Design review of the part built by this model. Coordinates are the model's own, in mm. Face numbers are marked on the shaded views. A direction names the side the tool comes from. Coordinates: 2 decimals unless noted, no trailing zeros. Loops run counter-clockwise (first coordinate to the right, second up) from the corner with the lowest first, then second, coordinate; pieces in that order, holes last. Notation, with made-up numbers: M -30.5,78 L -18.5,78 A12 ccw -18.5,92 Z; hole C 25,45 d5. An arc over 180 degrees is marked long. One line per item, written item: value.
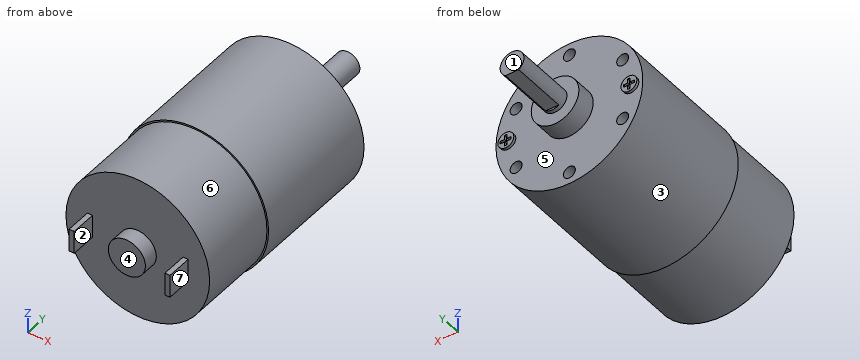
```python
from build123d import *

# Parameters (mm, degrees)
SKETCH1_R                 = 18.1
BASE_EXTRUDE_DEPTH        = 20
SKETCH2_R                 = 18.5
MOTOR_TOP_DEPTH           = 33.3
SKETCH3_R                 = 4.666403254
REAR_NUB_DEPTH            = 3.81
SKETCH4_W                 = 1.27
SKETCH4_H                 = 5.788702771
TEETH_PLUGS_DEPTH         = 6.35
SKETCH5_R                 = 6
AXLE_BASE_DEPTH           = 5
SKETCH7_R                 = 3
AXLE_DEPTH                = 15
SKETCH8_W                 = 0.5
SKETCH8_H                 = 14
D_SHAFT_CUTOUT_DEPTH      = 19.5
D_SHAFT_CUTOUT_DEPTH_BACK = 19.5
SKETCH9_R                 = 1.5
M3_SCREW_HOLES_DEPTH      = 10
SCREW_HOLE_PATTERN_COUNT  = 6
SKETCH10_R                = 2
PHILIPS_SCREWS_DEPTH      = 0.7


with BuildPart() as part:
    # Sketch1 → Base Extrude (new body)
    with BuildSketch(Plane(origin=(0, 0, 0), x_dir=(1, 0, 0), z_dir=(0, 1, 0))):
        Circle(SKETCH1_R)
    extrude(amount=BASE_EXTRUDE_DEPTH)

    # Sketch2 → Motor Top (add)
    with BuildSketch(Plane(origin=(0, 20, 0), x_dir=(1, 0, 0), z_dir=(0, 1, 0))):
        Circle(SKETCH2_R)
    extrude(amount=MOTOR_TOP_DEPTH)

    # Sketch3 → Rear nub (add)
    with BuildSketch(Plane.XZ):
        Circle(SKETCH3_R)
    extrude(amount=REAR_NUB_DEPTH)

    # Sketch4 → Teeth plugs (add)
    with BuildSketch(Plane.XZ):
        with Locations((-12.065, 0.236273582)):
            Rectangle(SKETCH4_W, SKETCH4_H)
        with Locations((12.065, 0.236273582)):
            Rectangle(SKETCH4_W, SKETCH4_H)
    extrude(amount=TEETH_PLUGS_DEPTH)

    # Sketch5 → Axle base (add)
    with BuildSketch(Plane(origin=(0, 53.3, 0), x_dir=(1, 0, 0), z_dir=(0, 1, 0))):
        Circle(SKETCH5_R)
    extrude(amount=AXLE_BASE_DEPTH)

    # Sketch7 → Axle (add)
    with BuildSketch(Plane(origin=(0, 58.3, 0), x_dir=(1, 0, 0), z_dir=(0, 1, 0))):
        Circle(SKETCH7_R)
    extrude(amount=AXLE_DEPTH)

    # Sketch8 → D shaft cutout (cut, two sides)
    with BuildSketch(Plane(origin=(0, 0, 0), x_dir=(0, 0, -1), z_dir=(1, 0, 0))) as d_shaft_cutout_sk:
        with Locations((2.75, 66.3)):
            Rectangle(SKETCH8_W, SKETCH8_H)
    extrude(amount=D_SHAFT_CUTOUT_DEPTH, mode=Mode.SUBTRACT)
    extrude(d_shaft_cutout_sk.sketch, amount=-D_SHAFT_CUTOUT_DEPTH_BACK, mode=Mode.SUBTRACT)

    # Sketch9 → M3 Screw Holes (cut)
    with BuildSketch(Plane(origin=(0, 53.3, 0), x_dir=(1, 0, 0), z_dir=(0, 1, 0))):
        with Locations((0, 15.5)):
            Circle(SKETCH9_R)
    m3_screw_holes = extrude(amount=-M3_SCREW_HOLES_DEPTH, mode=Mode.SUBTRACT)

    # Screw Hole Pattern: M3 Screw Holes ×6 about axis
    screw_hole_pattern_axis = Axis((0, 0, 0), (0, 1, 0))
    for i in range(1, SCREW_HOLE_PATTERN_COUNT):
        add(m3_screw_holes.rotate(screw_hole_pattern_axis, i * 360 / SCREW_HOLE_PATTERN_COUNT), mode=Mode.SUBTRACT)

    # Sketch10 → Philips Screws (add)
    with BuildSketch(Plane(origin=(0, 53.3, 0), x_dir=(1, 0, 0), z_dir=(0, 1, 0))):
        with Locations((-15.5, 0)):
            Circle(SKETCH10_R)
        Polygon((-16.943750133, -0.329942757), (-16.943750133, 0.329942757), (-15.829942757, 0.329942757), (-15.829942757, 1.40634253), (-15.170057243, 1.40634253), (-15.170057243, 0.329942757), (-14.166731925, 0.329942757), (-14.166731925, -0.329942757), (-15.170057243, -0.329942757), (-15.170057243, -1.370675678), (-15.829942757, -1.370675678), (-15.829942757, -0.329942757), align=None, mode=Mode.SUBTRACT)
        with Locations((15.5, 0)):
            Circle(SKETCH10_R)
        Polygon((15.829942757, 0.329942757), (16.943750133, 0.329942757), (16.943750133, -0.329942757), (15.829942757, -0.329942757), (15.829942757, -1.370675678), (15.170057243, -1.370675678), (15.170057243, -0.329942757), (14.166731925, -0.329942757), (14.166731925, 0.329942757), (15.170057243, 0.329942757), (15.170057243, 1.40634253), (15.829942757, 1.40634253), align=None, mode=Mode.SUBTRACT)
    extrude(amount=PHILIPS_SCREWS_DEPTH)


solid = part.part
```
(1) Tool access review of the marked faces 4, 5, 6 and 7: name each direction out of +Z, -Z, +X, -X, +Y, -Y from which nothing blocks a thin tool from reaching the whole face with its end or side.
Reply:
face 4: +Z, -Z, -Y
face 5: +Y
face 6: -Y
face 7: +Z, -Z, +X, -Y
(2) To check wall thickness, follow line 1 along Z through (x, y) = (0, 48.5); line 2 along Y through (x, z) = (6, 6); line 3 along X through (y, z) = (52.5, 8). State the ranges of each line that lie inside material, in increasing order. Write a range as [from, to].
Reply:
line 1: z = [-18.5, -17], [-14, 14], [17, 18.5]
line 2: y = [0, 53.3]
line 3: x = [-16.68, -14.9], [-11.94, 11.94], [14.9, 16.68]
(3) Insertion check: pin 1 (6 mm diameter, centred on y = 12, z = -10.5, fed in from +X); pin 2 (1 mm diameter, centred on y = 6.5, z = -1, fed in from -X); pin 3 (3.5 mm diameter, centred on x = -13, z = -8.5, fed in from +Y). Each pin has a flat end and moves straight along its axis. Give the tip position at first contact, or say it passes through.
Reply:
pin 1: stops at x = 16.47
pin 2: stops at x = -18.09
pin 3: stops at y = 53.3
(4) Mouldability with a two-part tool opening along X and no side actions: class the marked faces 1, 2 and 3 as released by +X, released by -X, zero draft, split by the parting line, or undercut.
Reply:
face 1: zero draft
face 2: undercut
face 3: split by the parting line
(5) We need section C-C on z = -7.75. State the section outline as (x, y) points.
Reply:
outline: M -16.8,20 L -16.36,20 L -16.36,0 L 16.36,0 L 16.36,20 L 16.8,20 L 16.8,53.3 L 14.92,53.3 L 14.92,43.3 L 11.92,43.3 L 11.92,53.3 L -11.92,53.3 L -11.92,43.3 L -14.92,43.3 L -14.92,53.3 L -16.8,53.3 Z
(6) We need section B-B on y = 45.5. State the section outline as (x, z) points.
Reply:
outline: C 0,0 d37; hole C -13.42,-7.75 d3; hole C -13.42,7.75 d3; hole C 0,-15.5 d3; hole C 0,15.5 d3; hole C 13.42,-7.75 d3; hole C 13.42,7.75 d3
(7) We need section D-D on y = 14. State the section outline as (x, z) points.
Reply:
outline: C 0,0 d36.2
